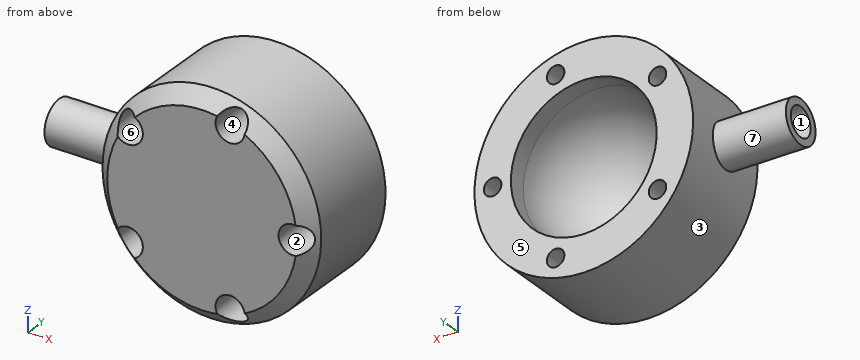
from build123d import *

# Parameters (mm, degrees)
BOSS_EXTRUDE1_REACH            = 92.554
BOSS_EXTRUDE1_END_RADIUS       = 30
SKETCH2_R                      = 6
CUT_EXTRUDE1_REACH             = 92.554
CUT_EXTRUDE1_END_RADIUS        = 20
SKETCH4_R                      = 4
CHAMFER1_SIZE                  = 4
CBORE_FOR_M4_SHCS1_D           = 4.8
CBORE_FOR_M4_SHCS1_CBORE_D     = 8
CBORE_FOR_M4_SHCS1_CBORE_DEPTH = 19


with BuildPart() as part:
    # Sketch1 → Revolve1 (revolve)
    with BuildSketch(Plane.XY, mode=Mode.PRIVATE) as revolve1_sk:
        with BuildLine():
            Line((20, 0), (20, -5))
            ThreePointArc((20, -5), (14.142135624, -19.142135624), (0, -25))
            Line((0, -25), (0, -30))
            Line((0, -30), (30, -30))
            Line((30, -30), (30, 0))
            Line((30, 0), (20, 0))
        make_face()
    revolve(revolve1_sk.sketch.rotate(Axis((0, 18.533057851, 0), (0, 1, 0)), 90), axis=Axis((0, 18.533057851, 0), (0, 1, 0)))

    # Boss-Extrude1: up to this cylinder (the profile starts outside it)
    boss_extrude1_end = Plane(origin=(0, -14, 0), z_dir=(0, -1, 0)) * Cylinder(BOSS_EXTRUDE1_END_RADIUS, 246.108, mode=Mode.PRIVATE)
    # Sketch2 → Boss-Extrude1 (add, up to the surface)
    with BuildSketch(Plane(origin=(-50, 0, 0), x_dir=(0, 0, -1), z_dir=(1, 0, 0)), mode=Mode.PRIVATE) as boss_extrude1_sk1:
        with Locations(Location((0, -14, 0), (0, 0, 180))):
            Circle(SKETCH2_R)
    boss_extrude1_tool1 = extrude(boss_extrude1_sk1.sketch, amount=BOSS_EXTRUDE1_REACH, mode=Mode.PRIVATE) - boss_extrude1_end
    add(boss_extrude1_tool1.solids().sort_by_distance((-50, -14, 0))[0])

    # Cut-Extrude1: up to this sphere (the profile starts outside it)
    cut_extrude1_end = Location((0, -5, 0)) * Sphere(CUT_EXTRUDE1_END_RADIUS, mode=Mode.PRIVATE)
    # Sketch4 → Cut-Extrude1 (cut, up to the surface)
    with BuildSketch(Plane.ZY.offset(50), mode=Mode.PRIVATE) as cut_extrude1_sk1:
        with Locations((0, -14)):
            Circle(SKETCH4_R)
    cut_extrude1_tool1 = extrude(cut_extrude1_sk1.sketch, amount=-CUT_EXTRUDE1_REACH, mode=Mode.PRIVATE) - cut_extrude1_end
    add(cut_extrude1_tool1.solids().sort_by_distance((-50, -14, 0))[0], mode=Mode.SUBTRACT)

    # Chamfer1
    chamfer1_edges = [part.edges().sort_by_distance(p)[0] for p in [
        (0, -30, 30),
    ]]
    chamfer(chamfer1_edges, length=CHAMFER1_SIZE)

    # CBORE for M4 SHCS1 (through all)
    with Locations(Plane(origin=(0, -30, 0), x_dir=(-1, 0, 0), z_dir=(0, -1, 0))):
        with Locations((-25, 0), (-7.725424859, -23.776412907), (20.225424859, -14.694631307), (20.225424859, 14.694631307), (-7.725424859, 23.776412907)):
            CounterBoreHole(CBORE_FOR_M4_SHCS1_D / 2, CBORE_FOR_M4_SHCS1_CBORE_D / 2, CBORE_FOR_M4_SHCS1_CBORE_DEPTH)


solid = part.part
Here's how the part is built. I have some questions about the finished solid (model axes, mm). Face numbers are marked on the shaded views. A direction names the side the tool comes from. Round coordinates to 2 decimals unless told otherwise and drop trailing zeros. Loops run counter-clockwise (first coordinate to the right, second up) from the corner with the lowest first, then second, coordinate; pieces in that order, holes last. Notation, with made-up numbers: M -7.5,27 L 12.5,27 A20 ccw 12.5,36 Z; hole C 49,33 d7. An arc over 180 degrees is marked long. Write each question's results on one line, items separated by ' | '. Start each with the question number.
(1) Will these pins go through, and if not, where does the flat tip stop? P1, Ø2, axis at y = -26.5, z = 14.5, coming from the +X side; P2, Ø10.5, axis at y = -14, z = 0, coming from the +X side; P3, Ø2.5, axis at x = 27, z = 0, coming from the -Y side; P4, Ø4, axis at x = 25, z = 0, coming from the -Y side.
(2) I want a section at B-B (y = -14). Please give me the cut outline in (x, z), then the cut area to 3 significant figures.
(3) I want a section at A-A (x = 0). Please give me the cut outline in (y, z), then the cut area to 3 significant figures.
(4) Thinking about a two-plate mould opening in X: for the marked faces 1, 2, 3 and 4, which applies, pulls with the +X half, pulls with the -X half, needs draft (parallel to the pull), parting line crosses it, or undercut?
(5) On a 3-axis mill with a long thin cutter (end or side, diameter ignored), from which of +Z, -Z, +X, -X, +Y, -Y can I reach the whole of each face in a straight line? I mean the marked faces 5, 6 and 7. Say none if no direction works.
(6) If I drill on probe 1 along Z at (x, y) = (6, -18); probe 2 along Z at (x, y) = (8.5, -19); probe 3 along X at (y, z) = (-4, 1), over which ranges is the centre line in solid material (lowest first)? Write a range as from..to.
(7) I want a section at C-C (y = -21). Please give me the cut outline in (x, z).
Solved:
1) P1: stops at x = 26.72 | P2: stops at x = 30 | P3: stops at y = -11 | P4: passes through
2) outline: M -50,-6 L -29.39,-6 A30 ccw long -29.39,6 L -50,6 L -50,4 L -17.41,4 A17.86 cw long -17.41,-4 L -50,-4 Z; hole C -20.23,-14.69 d8; hole C -20.23,14.69 d8; hole C 7.73,-23.78 d8; hole C 7.73,23.78 d8; hole C 25,0 d8 | area: 1,560 mm²
3) outline: M -30,-26 L -26,-30 L 0,-30 L 0,-20 L -5,-20 A20 cw -5,20 L 0,20 L 0,30 L -26,30 L -30,26 Z | area: 956 mm²
4) face 1: needs draft | face 2: undercut | face 3: parting line crosses it | face 4: undercut
5) face 5: +Z, -Z, +X, -X, +Y | face 6: -Y | face 7: -X
6) probe 1: z = -29.39..-27.39, -20.17..-13.96, 13.96..20.17, 27.39..29.39 | probe 2: z = -28.77..-27.7, -19.85..-11.48, 11.48..19.85, 27.7..28.77 | probe 3: x = -29.98..-19.97, 19.97..22.82, 27.18..29.98
7) outline: C 0,0 d60; hole C -20.23,-14.69 d8; hole C -20.23,14.69 d8; hole C 0,0 d24; hole C 7.73,-23.78 d8; hole C 7.73,23.78 d8; hole C 25,0 d8
